Autodesk Inventor part; units mm, degrees
ref_plane "Work Plane1" through (0, 0, -15) normal (0, 0, 1) x (1, 0, 0)
ref_plane "Work Plane2" through (0, 6, -14.6) normal (0, 0, 1) x (1, 0, 0)
ref_plane "Work Plane3" through (0, 6, -30) normal (0, -1, 0) x (1, 0, 0)
sketch "Sketch1" plane through (0, 0, 0) normal (1, 0, 0) x (0, 1, 0)
  line L0 (0, 0) -> (12, 0)
  line L1 (12, 0) -> (12, -30)
  line L2 (12, -30) -> (0, -30)
  line L3 (0, -30) -> (0, 0)
  circle A0 centre (6, -15) radius 0.4
  dimension "d0" = 30
  dimension "d1" = 12
  dimension "d2" = 6
  dimension "d3" = 15
  dimension "d4" = 0.8
extrude "Extrusion1" add sketch "Sketch1" against normal blind 50
ref_plane "Work Plane1" through (0, 0, -15) normal (0, 0, 1) x (1, 0, 0)
sketch "Sketch2" plane through (0, 0, 0) normal (0, 0, 1) x (1, 0, 0)
  line L0 (0, 0) -> (-50, 0)
  line L1 (0, 0) -> (0, 12)
  circle A0 centre (-10, 6) radius 3.2
  dimension "d7" = 6.4
  dimension "d8" = 6
  dimension "d9" = 10
extrude "Extrusion4" cut sketch "Sketch2" against normal blind 10.8
pattern_linear "Rectangular Pattern1" count 4 spacing 10 along (-1, 0, 0) of "Extrusion4"
ref_plane "Work Plane2" through (0, 6, -14.6) normal (0, 0, 1) x (1, 0, 0)
sketch "Sketch3" plane through (-10, 6, -10.8) normal (0, 0, 1) x (1, 0, 0)
  circle A0 centre (0, 0) radius 0.4
  circle A1 centre (0, 0) radius 3.2
  point P0 (10, -6)
  dimension "d20" = 0.8
extrude "Extrusion5" cut sketch "Sketch3" against normal blind 10 contours A0
pattern_linear "Rectangular Pattern2" count 4 spacing 10 along (-1, 0, 0) of "Extrusion5"
ref_plane "Work Plane3" through (0, 6, -30) normal (0, -1, 0) x (1, 0, 0)
sketch "Sketch4" plane through (0, 12, 0) normal (0, 1, 0) x (1, 0, 0)
  line L0 (0, 0) -> (0, 30)
  line L1 (0, 0) -> (-50, 0)
  circle A0 centre (-10, 7.4) radius 0.4
  circle A1 centre (-3.5, 3.5) radius 1.6
  dimension "d26" = 0.8
  dimension "d27" = 7.4
  dimension "d28" = 10
  dimension "d93" = 3.2
  dimension "d94" = 3.5
  dimension "d95" = 3.5
hole "Hole1" at (-10, 12, -7.4) direction (0, -1, 0) diameter 2.46 depth 7
pattern_linear "Rectangular Pattern4" count 4 spacing 10 along (-1, 0, 0) count 2 spacing 15.2 along (0, 0, -1) of "Hole1"
sketch "Sketch5" plane through (0, 0, -30) normal (0, 0, -1) x (-1, 0, 0)
  circle A0 centre (10, 6) radius 3.2
  line L0 (0, 12) -> (50, 12)
  line L1 (0, 12) -> (0, 0)
  dimension "d47" = 6.4
  dimension "d48" = 6
  dimension "d49" = 10
hole "Hole2" at (-10, 6, -30) direction (0, 0, 1) diameter 6.3 depth 10.8
pattern_linear "Rectangular Pattern5" count 4 spacing 10 along (-1, 0, 0) of "Hole2", "Extrusion4"
hole "Hole3" at (0, 6, -15) direction (-1, 0, 0) diameter 5.36 depth 7
sketch "Sketch6" plane through (-50, 0, 0) normal (-1, 0, 0) x (0, 0, 1)
  circle A0 centre (-15, 6) radius 2.15
  line L0 (-30, 0) -> (0, 0)
  dimension "d67" = 15
  dimension "d68" = 6
  dimension "d69" = 4.3
hole "Hole4" at (-50, 6, -15) direction (1, 0, 0) diameter 5.36 depth 7
hole "Hole5" at (-3.5, 12, -3.5) direction (0, -1, 0) diameter 3.2 end through all
pattern_linear "Rectangular Pattern6" count 2 spacing 43 along (-1, 0, 0) count 2 spacing 23 along (0, 0, -1) of "Hole5"
equation "\"d2\" = 0.5 * d1"
equation "\"d3\" = 0.5 * d0"
equation "\"d8\" = 0.5 * d1"
properties part number "Manifold_v4"
Could you check a few things on this model? Use its own coordinates, in mm. A direction names the side the tool comes from. Give positions to 0.01 mm unless a question says otherwise; leave off trailing zeros. Order: outer loops, then holes, each group sorted by start corner. A loop starts at its lowest first (then second) coordinate and runs counter-clockwise, first axis right, second up.
Q1. If I drill on line 1 along X through (y, z) = (6.25, -22.5); line 2 along X through (y, z) = (9.9, -7.4); line 3 along Y through (x, z) = (-30, -2.25), over which ranges is the centre line in solid material (lowest first)?
Q2. Suppose I cut it at D-D, the plane x = -6. Write out the boundary of the cut face in (y, z).
Q3. Suppose I cut it at A-A, the plane z = -26.5. Write out the boundary of the cut face in (x, y), and give its area (3 significant figures).
Q4. I'm going to push flat-ended pins straight in: P1, Ø5, axis at y = 6, z = -15, coming from the -X side; P2, Ø3, axis at x = -39, y = 5.5, coming from the +Z side; P3, Ø5, axis at y = 6, z = -15, coming from the +X side; P4, Ø2.5, axis at x = -46.5, z = -3.5, coming from the +Y side. Where does each tip first touch, or does it pass through?
Q5. We'd pull the mould along Y, two halves only. Please class faces 4 (the cylindrical face through (-10.694, 2.876, -5.324)), 5 (the cylindrical face through (-31.22, 10.46, -7.56)): +Y half, -Y half, draft (parallel to the pull), parting line (faces both ways), or undercut.
Q6. Suppose I cut it at B-B, the plane y = 10. Count the separate pieces of the cut face and the enclosed holes in it, and give its area (3 significant figures).
Q7. Suppose I cut it at C-C, the plane y = 1.5. Write out the boundary of the cut face in (x, z).
Q8. For faces 1 (the cylindrical face through (-21.22, 10.46, -7.56)), 2 (the cylindrical face through (-40.694, 2.876, -5.324)), 3 (the flat face through (-39, 6, -19.2)), which set-ups out of +Z, -Z, +X, -X, +Y, -Y let a thin tool reach every point of the face, with its end or its side?
Solution:
1. line 1: x = -50 to -43.14, -36.86 to -33.14, -26.86 to -23.14, -16.86 to -13.14, -6.86 to 0
1. line 2: x = -50 to -41.23, -38.77 to -31.23, -28.77 to -21.23, -18.77 to -11.23, -8.77 to 0
1. line 3: y = 0 to 2.8, 9.2 to 12
2. outline: (0, -30) - (12, -30) - (12, 0) - (0, 0) - close; hole circle Ø5.36 at (6, -15)
3. outline: (-50, 0) - (-48.1, 0) - (-48.1, 12) - (-50, 12) - close; (-44.9, 0) - (-5.1, 0) - (-5.1, 12) - (-44.9, 12) - close; (-1.9, 0) - (0, 0) - (0, 12) - (-1.9, 12) - close; hole circle Ø6.3 at (-40, 6); hole circle Ø6.3 at (-30, 6); hole circle Ø6.3 at (-20, 6); hole circle Ø6.3 at (-10, 6)
3. area: 399 mm2
4. P1: stops at x = -43
4. P2: stops at z = -10.8
4. P3: stops at x = -7
4. P4: passes through
5. face 4: undercut
5. face 5: draft
6. separate pieces: 1
6. enclosed holes: 12
6. area: 1,430 mm2
7. outline: (-50, -30) - (0, -30) - (0, 0) - (-50, 0) - close; hole circle Ø3.2 at (-46.5, -26.5); hole circle Ø3.2 at (-46.5, -3.5); hole circle Ø3.2 at (-3.5, -26.5); hole circle Ø3.2 at (-3.5, -3.5)
8. face 1: +Y
8. face 2: +Z
8. face 3: -Z
